from build123d import *

# Parameters (mm, degrees)
SKETCH3_R              = 20
BOSS_EXTRUDE3_DEPTH    = 3
F_10_24_TAPPED_HOLE1_D = 3.7973
SKETCH6_W              = 22.5
SKETCH6_H              = 12.2
CUT_EXTRUDE1_DEPTH     = 3
SKETCH7_R              = 1
SKETCH7_R_2            = 1.1
SKETCH7_R_3            = 1.122553576
CUT_EXTRUDE2_DEPTH     = 164.588932015


with BuildPart() as part:
    # Sketch3 → Boss-Extrude3 (new body)
    with BuildSketch(Plane(origin=(0, 0, 0), x_dir=(1, 0, 0), z_dir=(0, 1, 0))):
        with BuildLine():
            Line((-126.885775404, 33.210167511), (-126.885775404, -16.789832489))
            Line((-126.885775404, -16.789832489), (-84.87168845, -16.789832489))
            ThreePointArc((-84.87168845, -16.789832489), (-63.652193601, 16.862361112), (-30, 38.081855961))
            Line((-30, 38.081855961), (-30, -1.789832489))
            Line((-30, -1.789832489), (30, -1.789832489))
            Line((30, -1.789832489), (30, 38.081855961))
            ThreePointArc((30, 38.081855961), (63.652193601, 16.862361112), (84.87168845, -16.789832489))
            Line((84.87168845, -16.789832489), (126.885775404, -16.789832489))
            Line((126.885775404, -16.789832489), (126.885775404, 33.210167511))
            ThreePointArc((126.885775404, 33.210167511), (0, 103.210167511), (-126.885775404, 33.210167511))
        make_face()
        with Locations(Location((-96.223855306, 24.910723088, 0), (0, 0, 270))):
            Circle(SKETCH3_R, mode=Mode.SUBTRACT)
        with Locations(Location((96.223855306, 24.910723088, 0), (0, 0, 270))):
            Circle(SKETCH3_R, mode=Mode.SUBTRACT)
        with Locations(Location((-36.555626875, 67.506651026, 0), (0, 0, 270))):
            Circle(SKETCH3_R, mode=Mode.SUBTRACT)
        with Locations(Location((36.555626875, 67.506651026, 0), (0, 0, 270))):
            Circle(SKETCH3_R, mode=Mode.SUBTRACT)
    extrude(amount=BOSS_EXTRUDE3_DEPTH)

    # #10-24 Tapped Hole1 (through all)
    with Locations(Plane(origin=(0, 3, 0), x_dir=(1, 0, 0), z_dir=(0, 1, 0))):
        with Locations((-66.223855306, 24.910723088), (-96.223855306, 54.910723088), (-66.555626875, 67.506651026), (-6.555626875, 67.506651026), (6.555626875, 67.506651026), (66.555626875, 67.506651026), (96.223855306, 54.910723088), (66.223855306, 24.910723088)):
            Hole(F_10_24_TAPPED_HOLE1_D / 2)

    # Sketch6 → Cut-Extrude1 (cut)
    with BuildSketch(Plane.XZ):
        with Locations((6.85, -16.810167511)):
            Rectangle(SKETCH6_W, SKETCH6_H)
    extrude(amount=-CUT_EXTRUDE1_DEPTH, mode=Mode.SUBTRACT)

    # Sketch7 → Cut-Extrude2 (cut, through all)
    with BuildSketch(Plane.XZ):
        with Locations(Location((-13.053692885, -1.910723088, 0), (0, 0, 270))):
            Circle(SKETCH7_R)
        with Locations(Location((-19.702079803, -1.910723088, 0), (0, 0, 270))):
            Circle(SKETCH7_R)
        with Locations(Location((-13.053692885, -27.360397158, 0), (0, 0, 270))):
            Circle(SKETCH7_R)
        with Locations(Location((-4.804956753, -95.064096736, 0), (0, 0, 270))):
            Circle(SKETCH7_R)
        with Locations(Location((4.804956753, -95.064096736, 0), (0, 0, 270))):
            Circle(SKETCH7_R)
        with Locations(Location((-7.05, -16.810167511, 0), (0, 0, 270))):
            Circle(SKETCH7_R_2)
        with Locations(Location((20.754736903, -16.832218034, 0), (0, 0, 270))):
            Circle(SKETCH7_R_3)
    extrude(amount=-CUT_EXTRUDE2_DEPTH, mode=Mode.SUBTRACT)


solid = part.part
Source: CAD feature listing. Evaluate the final solid. Frame: model axes, mm. Round coordinates to 2 decimals unless told otherwise and drop trailing zeros. Loops run counter-clockwise (first coordinate to the right, second up) from the corner with the lowest first, then second, coordinate; pieces in that order, holes last.
Q1. Ray query, line 1 (X direction, y = 2.3, z = -37); line 2 (X direction, y = 2.25, z = -15); line 3 (X direction, y = 1.5, z = -51.5). Return the intervals inside material, ascending.
Q2. Section D-D, the plane z = 9. Return loops of the section in (x, y).
Q3. First-contact query: P1, Ø1.5, axis at x = -2.5, y = 2, coming from the +Z side; P2, Ø24, axis at x = -96.22, z = -24.91, coming from the -Y side; P3, Ø1.5, axis at y = 2, z = -67.5, coming from the -X side; P4, Ø1.5, axis at x = 8.5, y = 2, coming from the -Z side. Flat tips, straight axial feed; report the tip coordinate or a pass-through.
Q4. Mould query, pull axis Z, two halves, no side actions, for faces 1 (the face through (-2, 0, -44)), 2 (the face through (-82.707, 1.479, -39.652)), 3 (the face through (2.117, 1.479, -103.195)). Classes: pulls with the +Z half, pulls with the -Z half, needs draft (parallel to the pull), parting line crosses it, or undercut.
Q5. Section A-A, the plane x = -23. Return loops of the section in (y, z), plus the area to 3 significant figures.
Q6. Section C-C, the plane z = -81. Return loops of the section in (x, y), plus the area to 3 significant figures.
Q7. Section B-B, the plane y = 1.7. State how many separate pieces and enclosed holes the cut face has, plus the area to 3 significant figures.
Solutions:
1. line 1: x = -124.42 to -112.16, -80.29 to -32.9, -30 to 30, 32.9 to 80.29, 112.16 to 124.42
1. line 2: x = -126.89 to -113.6, -78.85 to -65.46, -30 to -4.4, 18.1 to 30, 65.46 to 78.85, 113.6 to 126.89
1. line 3: x = -113.31 to -48.55, -24.56 to 24.56, 48.55 to 113.31
2. outline: (-126.89, 0) - (-81.7, 0) - (-81.7, 3) - (-126.89, 3) - close; (81.7, 0) - (126.89, 0) - (126.89, 3) - (81.7, 3) - close
3. P1: stops at z = 1.79
3. P2: passes through
3. P3: stops at x = -98.02
3. P4: stops at z = -103.01
4. face 1: needs draft
4. face 2: undercut
4. face 3: pulls with the -Z half
5. outline: (0, -101.44) - (3, -101.44) - (3, -82.21) - (0, -82.21) - close; (0, -52.8) - (3, -52.8) - (3, 1.79) - (0, 1.79) - close
5. area: 221 mm2
6. outline: (-78.55, 0) - (-51.32, 0) - (-51.32, 3) - (-78.55, 3) - close; (-21.79, 0) - (21.79, 0) - (21.79, 3) - (-21.79, 3) - close; (51.32, 0) - (78.55, 0) - (78.55, 3) - (51.32, 3) - close
6. area: 294 mm2
7. separate pieces: 1
7. enclosed holes: 20
7. area: 15,000 mm2
